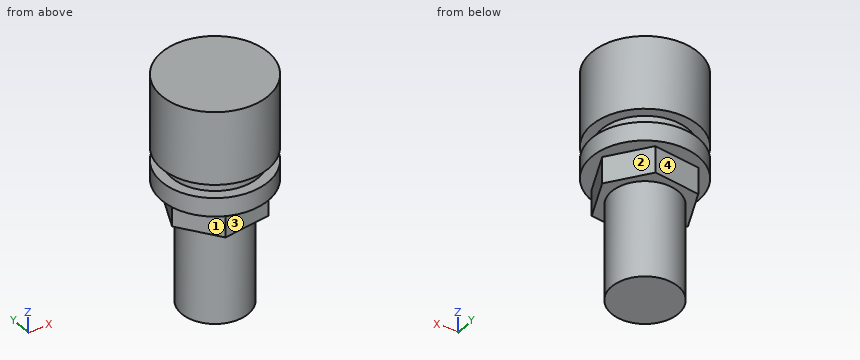
Autodesk Inventor part; units mm, degrees
ref_plane "YZ Plane" through (0, 0, 0) normal (1, 0, 0) x (0, 1, 0)
ref_plane "XZ Plane" through (0, 0, 0) normal (0, 1, 0) x (-1, 0, 0)
ref_plane "XY Plane" through (0, 0, 0) normal (0, 0, 1) x (1, 0, 0)
sketch "Sketch1" plane through (0, 0, 0) normal (0, 0, 1) x (1, 0, 0)
  circle A0 centre (0, 0) radius 8
  dimension "d0" = 16
extrude "Extrusion1" add sketch "Sketch1" along normal blind 11
sketch "Sketch2" plane through (0, 0, 0) normal (0, 0, -1) x (-1, 0, 0)
  circle A0 centre (0, 0) radius 6.5
  dimension "d3" = 13
extrude "Extrusion2" add sketch "Sketch2" along normal blind 2
sketch "Sketch3" plane through (0, 0, -2) normal (0, 0, -1) x (-1, 0, 0)
  circle A0 centre (0, 0) radius 8
  dimension "d6" = 16
extrude "Extrusion3" add sketch "Sketch3" along normal blind 2.8
sketch "Sketch4" plane through (0, 0, -4.8) normal (0, 0, -1) x (-1, 0, 0)
  line L0 (-2.7723, 6.3494) -> (4.1126, 5.5756)
  line L1 (4.1126, 5.5756) -> (6.8849, -0.7738)
  line L2 (6.8849, -0.7738) -> (2.7723, -6.3494)
  line L3 (2.7723, -6.3494) -> (-4.1126, -5.5756)
  line L4 (-4.1126, -5.5756) -> (-6.8849, 0.7738)
  line L5 (-6.8849, 0.7738) -> (-2.7723, 6.3494)
  point P0 (0, 0)
  point P1 (0, 0)
  dimension "d9" = 6
extrude "Extrusion4" add sketch "Sketch4" along normal blind 4
sketch "Sketch5" plane through (0, 0, -8.8) normal (0, 0, -1) x (-1, 0, 0)
  circle A0 centre (0, 0) radius 5
  dimension "d12" = 10
extrude "Extrusion5" add sketch "Sketch5" along normal blind 14.4
properties part number "HTC-30M_5x20mmFuse_Holder"
Verification items for the finished model (mm, model axes). Face numbers are marked on the shaded views. A direction names the side the tool comes from. Coordinates: 2 decimals unless noted, no trailing zeros. Loops run counter-clockwise (first coordinate to the right, second up) from the corner with the lowest first, then second, coordinate; pieces in that order, holes last. Notation, with made-up numbers: (-9, 48.5) -> (42, 48.5) arc R22 cw to (42, 74.5) -> close; hole circle Ø5 at (44, 36.5). An arc over 180 degrees is marked (long way). Put each result on its own line as item: value.
1. Section check C-C, the plane z = -5.5. Record the boundary of the cut face in (x, y), then the cut area to 3 significant figures.
Result set:
outline: (-6.88, -0.77) -> (-2.77, -6.35) -> (4.11, -5.58) -> (6.88, 0.77) -> (2.77, 6.35) -> (-4.11, 5.58) -> close
area: 125 mm^2
2. Section check D-D, the plane x = 0. Record the boundary of the cut face in (y, z).
Result set:
outline: (-8, -4.8) -> (-6.04, -4.8) -> (-6.04, -8.8) -> (-5, -8.8) -> (-5, -23.2) -> (5, -23.2) -> (5, -8.8) -> (6.04, -8.8) -> (6.04, -4.8) -> (8, -4.8) -> (8, -2) -> (6.5, -2) -> (6.5, 0) -> (8, 0) -> (8, 11) -> (-8, 11) -> (-8, 0) -> (-6.5, 0) -> (-6.5, -2) -> (-8, -2) -> close
3. Gauge pin test, flat end, axial feed: P1, Ø3, axis at y = 0.5, z = -13.5, coming from the +X side. Record the tip position at first contact, or that the pin passes through.
Result set:
P1: stops at x = 5
4. Tool access check on the marked faces 1, 2, 3 and 4. Record the directions out of +Z, -Z, +X, -X, +Y, -Y that give a thin tool (end or side, any length) a straight path to the whole face; none if there is none.
Result set:
face 1: -Z, -X, -Y
face 2: -Z, +X, +Y
face 3: -Z, +X, -Y
face 4: -Z, -X, +Y
5. Section check B-B, the plane y = -2.5. Record the boundary of the cut face in (x, z), then the cut area to 3 significant figures.
Result set:
outline: (-7.6, -4.8) -> (-5.61, -4.8) -> (-5.61, -8.8) -> (-4.33, -8.8) -> (-4.33, -23.2) -> (4.33, -23.2) -> (4.33, -8.8) -> (5.46, -8.8) -> (5.46, -4.8) -> (7.6, -4.8) -> (7.6, -2) -> (6, -2) -> (6, 0) -> (7.6, 0) -> (7.6, 11) -> (-7.6, 11) -> (-7.6, 0) -> (-6, 0) -> (-6, -2) -> (-7.6, -2) -> close
area: 403 mm^2
6. Thickness scan on line 1 (Z direction, x = -7, y = 3.75); line 2 (X direction, y = 0.25, z = -19); line 3 (Z direction, x = -5.25, y = 0.75). Record the ranges inside material, lowest first.
Result set:
line 1: z = -4.8 to -2, 0 to 11
line 2: x = -4.99 to 4.99
line 3: z = -8.8 to 11
7. Section check A-A, the plane y = 7.25. Record the boundary of the cut face in (x, z), then the cut area to 3 significant figures.
Result set:
outline: (-3.38, -4.8) -> (3.38, -4.8) -> (3.38, -2) -> (-3.38, -2) -> close; (-3.38, 0) -> (3.38, 0) -> (3.38, 11) -> (-3.38, 11) -> close
area: 93.3 mm^2
